from build123d import *

# Parameters (mm, degrees)
F1_DEPTH = 151.5


with BuildPart() as f1:
    # F0 (on Front) → F1 (new body)
    with BuildSketch(Plane.XZ):
        Polygon((0.75, 48), (0, 48), (-0.75, 48), (-1.5, 8), (-8.5, 8), (-9.25, 48), (-10, 48), (-10.75, 48), (-11.5, 8), (-18.5, 8), (-19.25, 48), (-20, 48), (-20.75, 48), (-21.5, 8), (-28.5, 8), (-29.25, 48), (-30, 48), (-30.75, 48), (-31.5, 8), (-38.5, 8), (-39.25, 48), (-40, 48), (-40.75, 48), (-41.5, 8), (-48.5, 8), (-49.25, 48), (-50, 48), (-50.75, 48), (-51.5, 8), (-58.5, 8), (-59.25, 48), (-60, 48), (-60.75, 48), (-61.5, 8), (-68.5, 8), (-69.25, 48), (-70, 48), (-70.75, 48), (-71.5, 8), (-78.5, 8), (-79.25, 48), (-80, 48), (-80.75, 48), (-81.5, 8), (-88.5, 8), (-89.25, 48), (-90, 48), (-90.75, 48), (-91.5, 8), (-98.5, 8), (-99.25, 48), (-100, 48), (-100.75, 48), (-101.5, 8), (-108.5, 8), (-109.25, 48), (-110, 48), (-110.75, 48), (-111.5, 8), (-118.5, 8), (-119.25, 48), (-120, 48), (-120.75, 48), (-121.5, 8), (-128.5, 8), (-129.25, 48), (-130, 48), (-130.75, 48), (-131.5, 8), (-141, 8), (-141, 48.199648), (-145, 48.199648), (-145, 0), (155, 0), (155, 48), (151, 48), (151, 8), (141.5, 8), (140.75, 48), (140, 48), (139.25, 48), (138.5, 8), (131.5, 8), (130.75, 48), (130, 48), (129.25, 48), (128.5, 8), (121.5, 8), (120.75, 48), (120, 48), (119.25, 48), (118.5, 8), (111.5, 8), (110.75, 48), (110, 48), (109.25, 48), (108.5, 8), (101.5, 8), (100.75, 48), (100, 48), (99.25, 48), (98.5, 8), (91.5, 8), (90.75, 48), (90, 48), (89.25, 48), (88.5, 8), (81.5, 8), (80.75, 48), (80, 48), (79.25, 48), (78.5, 8), (71.5, 8), (70.75, 48), (70, 48), (69.25, 48), (68.5, 8), (61.5, 8), (60.75, 48), (60, 48), (59.25, 48), (58.5, 8), (51.5, 8), (50.75, 48), (50, 48), (49.25, 48), (48.5, 8), (41.5, 8), (40.75, 48), (40, 48), (39.25, 48), (38.5, 8), (31.5, 8), (30.75, 48), (30, 48), (29.25, 48), (28.5, 8), (21.5, 8), (20.75, 48), (20, 48), (19.25, 48), (18.5, 8), (11.5, 8), (10.75, 48), (10, 48), (9.25, 48), (8.5, 8), (1.5, 8), align=None)
    extrude(amount=F1_DEPTH)


solid = f1.part
Check sheet for the modelled part. Datum: model origin and axes. Units: mm. Give positions to 0.01 mm unless a question says otherwise; leave off trailing zeros. Return JSON: item names as keys, results as strings. Group by question number.
1. Go/stop test with flat-tipped pins: pin 1 (1.6 mm diameter, centred on x = -120, y = -47.5, fed in from +Z); pin 2 (5.5 mm diameter, centred on x = 115, y = -94, fed in from +Z). Record where each tip stops, or that it passes through.
2. Cross-section at A-A on z = 40. State how many separate pieces and enclosed holes the cut face has, plus the area to 3 significant figures.
3. Thickness scan on L1, parallel to Z at x = -4, y = -132.5; L2, parallel to Z at x = -50, y = -69.5. Record the ranges inside material, lowest first.
Return value:
{
 "1": {"pin 1": "z = 48", "pin 2": "z = 8"},
 "2": {"separate pieces": "30", "enclosed holes": "0", "area": "8,850 mm^2"},
 "3": {"L1": "0 to 8", "L2": "0 to 48"}
}
